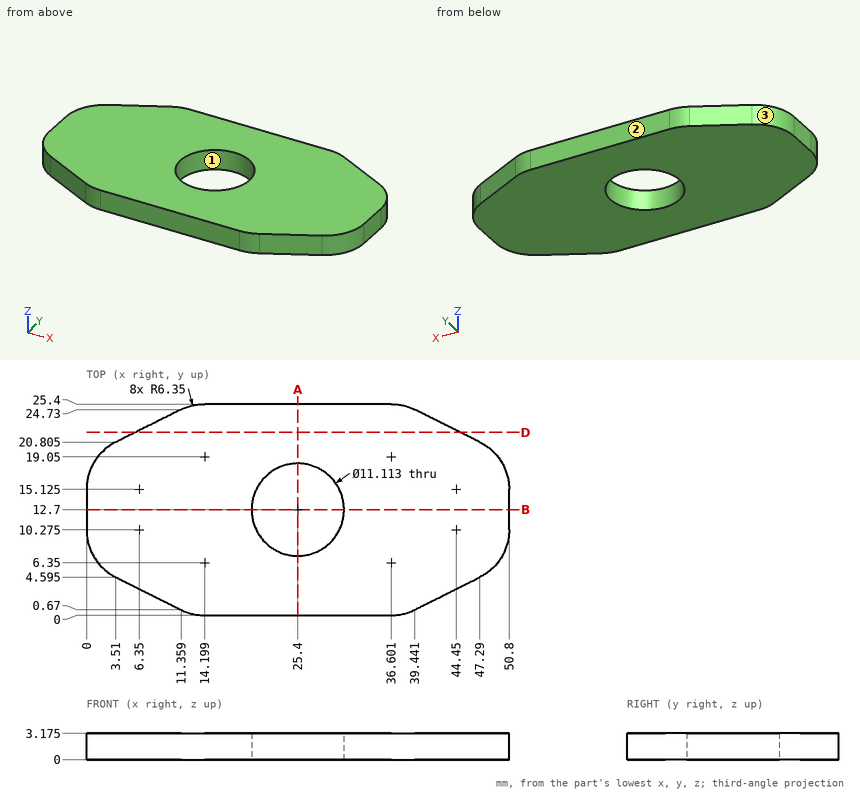
Check sheet for the drawn part. Datum: minimum x, y, z corner. Units: mm. Give positions to 0.01 mm unless a question says otherwise; leave off trailing zeros. Order: outer loops, then holes, each group sorted by start corner. A loop starts at its lowest first (then second) coordinate and runs counter-clockwise, first axis right, second up. Notation, with made-up numbers: (80.5, 39.25) - (108.5, 39.25) arc R24 cw to (108.5, 55.25) - close; hole circle Ø2 at (46.5, 12). An arc over 180 degrees is marked (long way). Answer as a JSON object with one key per item and string values.
(1) Draft check along X on the marked faces 1, 2 and 3. Enter one of: released by +X, released by -X, zero draft, split by the parting line, or undercut.
Report:
{"face 1": "undercut", "face 2": "zero draft", "face 3": "released by -X"}
(2) Material ranges on line 1 (Y direction, x = 25.4, z = 2.15); line 2 (X direction, y = 7.75, z = 2.15) (1 decimal); line 3 (Y direction, x = 24.5, z = 0.8), recorded low to high.
Report:
{"line 1": "0 to 7.14, 18.26 to 25.4", "line 2": "0.5 to 22.9, 27.9 to 50.3", "line 3": "0 to 7.22, 18.18 to 25.4"}
(3) Depth check by flat-ended pin: pin 1 Ø6.5 at (x, y) = (25.4, 12.7) entering from +Z. Enter the tip coordinate at first touch or a pass-through.
Report:
{"pin 1": "through"}
(4) Cross-section at B-B (y = 12.7). Record the cut outline in (x, z) (1 decimal).
Report:
{"outline": "(0, 0) - (19.8, 0) - (19.8, 3.2) - (0, 3.2) - close; (31, 0) - (50.8, 0) - (50.8, 3.2) - (31, 3.2) - close"}
(5) Cross-section at A-A (x = 25.4). Record the cut outline in (y, z) (1 decimal).
Report:
{"outline": "(0, 0) - (7.1, 0) - (7.1, 3.2) - (0, 3.2) - close; (18.3, 0) - (25.4, 0) - (25.4, 3.2) - (18.3, 3.2) - close"}
(6) Cross-section at D-D (y = 22). Record the cut outline in (x, z) (1 decimal), then the cut area to 3 significant figures.
Report:
{"outline": "(5.9, 0) - (44.9, 0) - (44.9, 3.2) - (5.9, 3.2) - close", "area": "124 mm^2"}
